Model file for the job. Use its own axes, mm. Coordinates: 2 decimals unless noted, no trailing zeros. Order: outer loops, then holes, each group sorted by start corner. A loop starts at its lowest first (then second) coordinate and runs counter-clockwise, first axis right, second up. Notation, with made-up numbers: (9, 54.25) -> (52, 54.25) arc R15 cw to (52, 67.25) -> close; hole circle Ø5 at (-38, -37). An arc over 180 degrees is marked (long way). Write item = value, one per line. Start each with the question number.
Q1. Cut at A-A, the plane x = 43.5. List the corners of the cut face in (y, z), plus the area to 3 significant figures.
Q2. Cut at B-B, the plane z = 1.75. List the corners of the cut face in (x, y), plus the area to 3 significant figures.
Q3. Cut at C-C, the plane y = 7.5. List the corners of the cut face in (x, z).
Q4. Wall check: line 1 (Z direction, x = 27.5, y = 10.25); line 2 (Y direction, x = -17.5, z = 0.25). Give the ranges that are in metal, low to high. Write a range as from..to.
Q5. Flat gauge pins, fed straight in: pin 1 (6 mm diameter, centred on x = 13, y = 6.5, fed in from +Z); pin 2 (0.9 mm diameter, centred on x = 21, z = 0, fed in from -Y); pin 3 (4 mm diameter, centred on y = 2.5, z = -0.5, fed in from -X). Where does each tip first touch, or does it go through?
from build123d import *

# Parameters (mm, degrees)
SKETCH_1_R      = 0.4
EXTRUDE_1_DEPTH = 10
SKETCH_2_W      = 100
SKETCH_2_H      = 0.8
EXTRUDE_2_DEPTH = 0.8
FILLET_1_R      = 0.4
SKETCH_3_R      = 0.4
EXTRUDE_3_DEPTH = 5
SKETCH_4_R      = 0.4
EXTRUDE_4_DEPTH = 5
CHAMFER_1_SIZE  = 0.4


with BuildPart() as part:
    # 草图1 → 凸台-拉伸1 (new body)
    with BuildSketch(Plane(origin=(0, 0, 0), x_dir=(1, 0, 0), z_dir=(0, 1, 0))):
        with Locations(Location((0, 0, 0), (0, 0, 270))):
            Circle(SKETCH_1_R)
    extrude(amount=EXTRUDE_1_DEPTH)

    # 草图2 → 凸台-拉伸2 (add)
    with BuildSketch(Plane(origin=(0, 10, 0), x_dir=(1, 0, 0), z_dir=(0, 1, 0))):
        Rectangle(SKETCH_2_W, SKETCH_2_H)
    extrude(amount=EXTRUDE_2_DEPTH)

    # 圆角1
    fillet_1_edges = [part.edges().sort_by_distance(p)[0] for p in [
        (50, 10, 0),
        (50, 10.8, 0),
        (-50, 10, 0),
        (-50, 10.8, 0),
    ]]
    fillet(fillet_1_edges, radius=FILLET_1_R - 0.0001)  # a hair under: the kernel refuses the full size

    # 草图3 → 凸台-拉伸3 (add)
    with BuildSketch(Plane.XY.offset(0.4)):
        with Locations((49.6, 10.4)):
            Circle(SKETCH_3_R)
    extrude(amount=EXTRUDE_3_DEPTH)

    # 草图4 → 凸台-拉伸4 (add)
    with BuildSketch(Plane(origin=(0, 0, -0.4), x_dir=(-1, 0, 0), z_dir=(0, 0, -1))):
        with Locations((49.6, 10.4)):
            Circle(SKETCH_4_R)
    extrude(amount=EXTRUDE_4_DEPTH)

    # 倒角1
    chamfer_1_edges = [part.edges().sort_by_distance(p)[0] for p in [
        (49.2, 10.4, 5.4),
        (-49.2, 10.4, -5.4),
    ]]
    chamfer(chamfer_1_edges, length=CHAMFER_1_SIZE)


solid = part.part
Here are the results:
q1.outline = (10, -0.4) -> (10.8, -0.4) -> (10.8, 0.4) -> (10, 0.4) -> close
q1.area = 0.640 mm²
q2.outline = circle Ø0.8 at (49.6, 10.4)
q2.area = 0.503 mm²
q3.outline = circle Ø0.8 at (0, 0)
q4.line_1 = -0.4..0.4
q4.line_2 = 10..10.8
q5.pin_1 = through
q5.pin_2 = 10
q5.pin_3 = -0.4
